from build123d import *

# Parameters (mm, degrees)
F0_W     = 72.195024
F0_H     = 71.365238
F1_DEPTH = 76.2
F2_SIZE  = 5.08
F3_R     = 10.044016
F3_R_2   = 9.812081
F4_DEPTH = 76.2
F6_DEPTH = 50.8


with BuildPart() as f1:
    # F0 (on Front) → F1 (new body)
    with BuildSketch(Plane.XZ):
        Rectangle(F0_W, F0_H)
    extrude(amount=F1_DEPTH)

    # F2
    f2_edges = [f1.edges().sort_by_distance(p)[0] for p in [
        (0, -76.2, -35.682619),
        (36.097512, -76.2, 0),
        (0, -76.2, 35.682619),
        (-36.097512, -76.2, 0),
        (36.097512, -38.1, -35.682619),
        (36.097512, -38.1, 35.682619),
        (36.097512, 0, 0),
        (-36.097512, -38.1, 35.682619),
        (0, 0, 35.682619),
        (-36.097512, -38.1, -35.682619),
        (-36.097512, 0, 0),
        (0, 0, -35.682619),
    ]]
    chamfer(f2_edges, length=F2_SIZE)

    # F3 (on Front) → F4 (cut)
    with BuildSketch(Plane.XZ):
        with Locations((-17.218977, 18.048741)):
            Circle(F3_R)
        with Locations((17.218918, 19.29348)):
            Circle(F3_R_2)
    extrude(amount=F4_DEPTH, mode=Mode.SUBTRACT)

    # F5 (on Front) → F6 (join)
    with BuildSketch(Plane.XZ):
        Polygon((11.202648, -24.528347), (11.202648, -8.249946), (-4.279031, -3.219644), (-13.847235, -16.389146), (-4.279031, -29.558649), align=None)
    extrude(amount=-F6_DEPTH)


solid = f1.part
Can you work these out from the model? Positions are in its coordinate system, mm. A direction names the side the tool comes from. Give positions to 0.01 mm unless a question says otherwise; leave off trailing zeros. Order: outer loops, then holes, each group sorted by start corner. A loop starts at its lowest first (then second) coordinate and runs counter-clockwise, first axis right, second up. Notation, with made-up numbers: M 26.25,-24.5 L 71.25,-24.5 A21 cw 71.25,13.5 Z; hole C 14.5,6 d9. An arc over 180 degrees is marked long. Use one line per item in the form item = value. Start each with the question number.
Item 1: If I drill on line 1 along X through (y, z) = (-40, 12); line 2 along Y through (x, z) = (-27, 30); line 3 along X through (y, z) = (-16, 20), over which ranges is the centre line in solid material (lowest first)?
Item 2: If we section it at D-D (y = 24.5): Write out the boundary of the cut face in (x, z).
Item 3: If we section it at B-B (y = -59): Write out the boundary of the cut face in (x, z).
Item 4: If we section it at A-A (x = -19.5): Write out the boundary of the cut face in (y, z).
Item 5: Will these pins go through, and if not, where does the flat tip stop? pin 1 Ø6 at (y, z) = (19, -20) entering from +X; pin 2 Ø16 at (x, z) = (-17.22, 18.05) entering from -Y; pin 3 Ø10 at (x, z) = (-8, 23.5) entering from +Y.
Item 6: If we section it at C-C (z = 12): Write out the boundary of the cut face in (x, y), then the cut area to 3 significant figures.
Item 7: For faces 1 (the flat face through (11.203, 25, -17)), 2 (the flat face through (3.57, 25.04, -5.77)), 3 (the flat face through (32.958, -72.726, -32.137)), which set-ups out of +Z, -Z, +X, -X, +Y, -Y let a thin tool reach every point of the face, with its end or its side?
Outcome:
q1.line_1 = -36.1 to -25.24, -9.2 to 10.66, 23.78 to 36.1
q1.line_2 = -76.2 to 0
q1.line_3 = -36.1 to -27.07, -7.37 to 7.43, 27.01 to 36.1
q2.outline = M -13.85,-16.39 L -4.28,-29.56 L 11.2,-24.53 L 11.2,-8.25 L -4.28,-3.22 Z
q3.outline = M -36.1,-30.6 L -31.02,-35.68 L 31.02,-35.68 L 36.1,-30.6 L 36.1,30.6 L 31.02,35.68 L -31.02,35.68 L -36.1,30.6 Z; hole C -17.22,18.05 d20.09; hole C 17.22,19.29 d19.62
q4.outline = M -76.2,-30.6 L -71.12,-35.68 L -5.08,-35.68 L 0,-30.6 L 0,8.27 L -76.2,8.27 Z; M -76.2,27.83 L 0,27.83 L 0,30.6 L -5.08,35.68 L -71.12,35.68 L -76.2,30.6 Z
q5.pin_1 = 11.2
q5.pin_2 = through
q5.pin_3 = 0
q6.outline = M -36.1,-71.12 L -31.02,-76.2 L -25.24,-76.2 L -25.24,0 L -31.02,0 L -36.1,-5.08 Z; M -9.2,-76.2 L 10.66,-76.2 L 10.66,0 L -9.2,0 Z; M 23.78,-76.2 L 31.02,-76.2 L 36.1,-71.12 L 36.1,-5.08 L 31.02,0 L 23.78,0 Z
q6.area = 3,230 mm2
q7.face_1 = +Z, -Z, +X, +Y
q7.face_2 = +Z, +X, +Y
q7.face_3 = -Z, +X, -Y
